The model under review builds one solid part; all positions refer to its coordinate system, in mm. Round coordinates to 2 decimals unless told otherwise and drop trailing zeros. Loops run counter-clockwise (first coordinate to the right, second up) from the corner with the lowest first, then second, coordinate; pieces in that order, holes last. Notation, with made-up numbers: M -16,-30 L 24,-30 A13 cw 24,-17 Z; hole C 32,55 d5. An arc over 180 degrees is marked long. Return JSON: item names as keys, results as strings. Group by question number.
Q1. Clearance check with flat-ended pins moving along their axes: pin 1 Ø5 at (x, z) = (1.5, 57.5) entering from +Y; pin 2 Ø2 at (y, z) = (-2, 55) entering from -X. State where each tip first meets the part, or that it passes through.
Q2. Consider section C-C (x = 10). State the section outline as (y, z) points.
Q3. Consider section A-A (x = 0). State the section outline as (y, z) points, and give its area (3 significant figures).
Q4. To check wall thickness, follow line 1 along X through (y, z) = (4.25, 45.5); line 2 along Y through (x, z) = (-10, 80). State the ranges of each line that lie inside material, in increasing order.
Autodesk Inventor part; units mm, degrees
ref_plane "YZ Plane" through (0, 0, 0) normal (1, 0, 0) x (0, 1, 0)
ref_plane "XZ Plane" through (0, 0, 0) normal (0, 1, 0) x (-1, 0, 0)
ref_plane "XY Plane" through (0, 0, 0) normal (0, 0, 1) x (1, 0, 0)
feature "ソリッド1" [suppressed]
sketch "スケッチ2" plane through (0, 0, 0) normal (0, 0, 1) x (1, 0, 0)
  line L0 (-12.5, 5.15) -> (-7, 5.15)
  line L1 (-7, 5.15) -> (-7, 3.15)
  line L2 (-7, 3.15) -> (-4.5, 3.15)
  line L3 (-4.5, 3.15) -> (-4.5, -3.15)
  line L4 (-4.5, -3.15) -> (-7, -3.15)
  line L5 (-7, -3.15) -> (-7, -5.15)
  line L6 (-7, -5.15) -> (-12.5, -5.15)
  line L7 (-12.5, -5.15) -> (-12.5, -3.15)
  line L8 (-12.5, -3.15) -> (-15, -3.15)
  line L9 (-15, -3.15) -> (-15, -14)
  arc A0 (-15, -14) -> (-14, -15) centre (-14, -14) ccw
  line L10 (-14, -15) -> (-3.15, -15)
  line L11 (-3.15, -15) -> (-3.15, -12.5)
  line L12 (-3.15, -12.5) -> (-5.15, -12.5)
  line L13 (-5.15, -12.5) -> (-5.15, -7)
  line L14 (-5.15, -7) -> (-3.15, -7)
  line L15 (-3.15, -7) -> (-3.15, -4.5)
  line L16 (-3.15, -4.5) -> (3.15, -4.5)
  line L17 (3.15, -4.5) -> (3.15, -7)
  line L18 (3.15, -7) -> (5.15, -7)
  line L19 (5.15, -7) -> (5.15, -12.5)
  line L20 (5.15, -12.5) -> (3.15, -12.5)
  line L21 (3.15, -12.5) -> (3.15, -15)
  line L22 (3.15, -15) -> (14, -15)
  arc A1 (14, -15) -> (15, -14) centre (14, -14) ccw
  line L23 (15, -14) -> (15, -3.15)
  line L24 (15, -3.15) -> (12.5, -3.15)
  line L25 (12.5, -3.15) -> (12.5, -5.15)
  line L26 (12.5, -5.15) -> (7, -5.15)
  line L27 (7, -5.15) -> (7, -3.15)
  line L28 (7, -3.15) -> (4.5, -3.15)
  line L29 (4.5, -3.15) -> (4.5, 3.15)
  line L30 (4.5, 3.15) -> (7, 3.15)
  line L31 (7, 3.15) -> (7, 5.15)
  line L32 (7, 5.15) -> (12.5, 5.15)
  line L33 (12.5, 5.15) -> (12.5, 3.15)
  line L34 (12.5, 3.15) -> (15, 3.15)
  line L35 (15, 3.15) -> (15, 14)
  arc A2 (15, 14) -> (14, 15) centre (14, 14) ccw
  line L36 (14, 15) -> (3.15, 15)
  line L37 (3.15, 15) -> (3.15, 12.5)
  line L38 (3.15, 12.5) -> (5.15, 12.5)
  line L39 (5.15, 12.5) -> (5.15, 7)
  line L40 (5.15, 7) -> (3.15, 7)
  line L41 (3.15, 7) -> (3.15, 4.5)
  line L42 (3.15, 4.5) -> (-3.15, 4.5)
  line L43 (-3.15, 4.5) -> (-3.15, 7)
  line L44 (-3.15, 7) -> (-5.15, 7)
  line L45 (-5.15, 7) -> (-5.15, 12.5)
  line L46 (-5.15, 12.5) -> (-3.15, 12.5)
  line L47 (-3.15, 12.5) -> (-3.15, 15)
  line L48 (-3.15, 15) -> (-14, 15)
  arc A3 (-14, 15) -> (-15, 14) centre (-14, 14) ccw
  line L49 (-15, 14) -> (-15, 3.15)
  line L50 (-15, 3.15) -> (-12.5, 3.15)
  line L51 (-12.5, 3.15) -> (-12.5, 5.15)
  circle A4 centre (10, 10) radius 3
  circle A5 centre (-10, 10) radius 3
  circle A6 centre (-10, -10) radius 3
  circle A7 centre (10, -10) radius 3
  circle A8 centre (0, 0) radius 2.5
extrude "押し出し1" add sketch "スケッチ2" along normal blind 165
equation "\"d1\" = L"
equation "\"L\" = 165"
properties part number "AFS-3030-200"
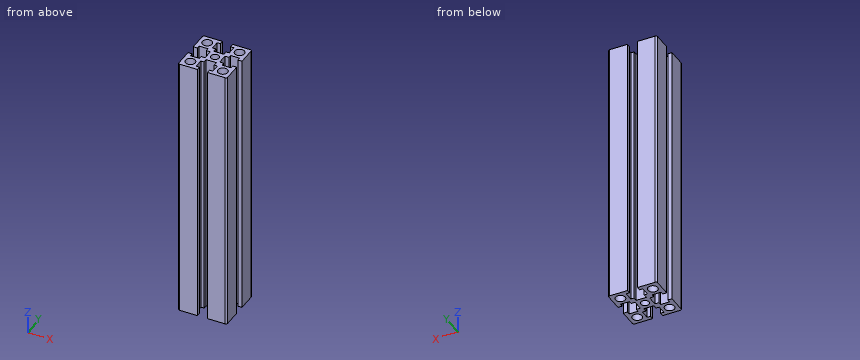
Values:
{
 "1": {"pin 1": "stops at y = 15", "pin 2": "stops at x = -4.5"},
 "2": {"outline": "M -15,0 L -13,0 L -13,165 L -15,165 Z; M -7,0 L -5.15,0 L -5.15,165 L -7,165 Z; M 5.15,0 L 7,0 L 7,165 L 5.15,165 Z; M 13,0 L 15,0 L 15,165 L 13,165 Z"},
 "3": {"outline": "M -4.5,0 L -2.5,0 L -2.5,165 L -4.5,165 Z; M 2.5,0 L 4.5,0 L 4.5,165 L 2.5,165 Z", "area": "660 mm2"},
 "4": {"line 1": "x = -15 to -12.5, -7 to 7, 12.5 to 15", "line 2": "y = -15 to -13, -7 to -5.15, 5.15 to 7, 13 to 15"}
}
